```python
from build123d import *

# Parameters (mm, degrees)
SKETCH1_R           = 1.6
BOSS_EXTRUDE1_DEPTH = 2


with BuildPart() as part:
    # Sketch1 → Boss-Extrude1 (new body)
    with BuildSketch(Plane.XY):
        with BuildLine():
            Line((-42, 25.469603275), (-57, 25.469603275))
            Line((-57, 25.469603275), (-57, -22.030396725))
            ThreePointArc((-57, -22.030396725), (-56.121320344, -24.151717068), (-54, -25.030396725))
            Line((-54, -25.030396725), (54, -25.030396725))
            ThreePointArc((54, -25.030396725), (56.121320344, -24.151717068), (57, -22.030396725))
            Line((57, -22.030396725), (57, 25.469603275))
            Line((57, 25.469603275), (42, 25.469603275))
            Line((42, 25.469603275), (42, 55.969603275))
            ThreePointArc((42, 55.969603275), (41.121320344, 58.090923619), (39, 58.969603275))
            Line((39, 58.969603275), (7, 58.969603275))
            Line((7, 58.969603275), (7, 43.469603275))
            Line((7, 43.469603275), (-7, 43.469603275))
            Line((-7, 43.469603275), (-7, 58.969603275))
            Line((-7, 58.969603275), (-39, 58.969603275))
            ThreePointArc((-39, 58.969603275), (-41.121320344, 58.090923619), (-42, 55.969603275))
            Line((-42, 55.969603275), (-42, 25.469603275))
        make_face()
        with Locations((54, -22.030396725)):
            Circle(SKETCH1_R, mode=Mode.SUBTRACT)
        with Locations(Location((-54, -22.030396725, 0), (0, 0, 180))):
            Circle(SKETCH1_R, mode=Mode.SUBTRACT)
        with Locations((39, 55.969603275)):
            Circle(SKETCH1_R, mode=Mode.SUBTRACT)
        with Locations(Location((-39, 55.969603275, 0), (0, 0, 180))):
            Circle(SKETCH1_R, mode=Mode.SUBTRACT)
    extrude(amount=BOSS_EXTRUDE1_DEPTH)


solid = part.part
```
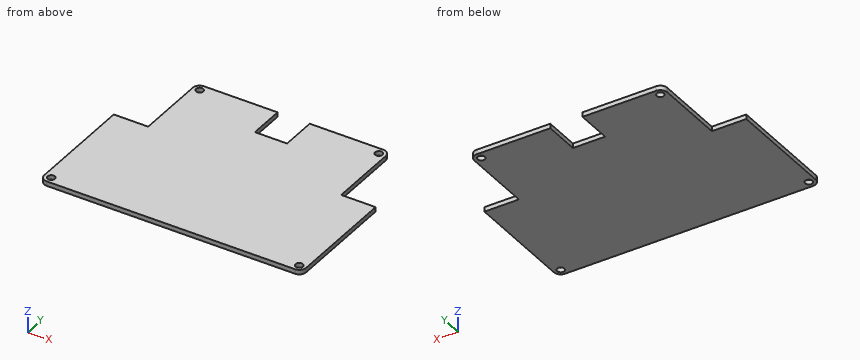
Could you check a few things on this model? Use its own coordinates, in mm. Round coordinates to 2 decimals unless told otherwise and drop trailing zeros. Loops run counter-clockwise (first coordinate to the right, second up) from the corner with the lowest first, then second, coordinate; pieces in that order, holes last. Notation, with made-up numbers: M 44,-4.5 L 93,-4.5 A11 cw 93,1.5 Z; hole C -8.75,56 d2. An arc over 180 degrees is marked long. Answer as CSV lines item,"result".
1) Imagine slicing it at A-A on z = 1. List the corners of the cut face in (x, y) for me, and give its area (3 significant figures).
From the geometry:
outline,"M -57,-22.03 A3 ccw -54,-25.03 L 54,-25.03 A3 ccw 57,-22.03 L 57,25.47 L 42,25.47 L 42,55.97 A3 ccw 39,58.97 L 7,58.97 L 7,43.47 L -7,43.47 L -7,58.97 L -39,58.97 A3 ccw -42,55.97 L -42,25.47 L -57,25.47 Z; hole C -54,-22.03 d3.2; hole C -39,55.97 d3.2; hole C 39,55.97 d3.2; hole C 54,-22.03 d3.2"
area,"8,310 mm^2"
2) If I drill on probe 1 along X at (y, z) = (46, 1.75); probe 2 along Y at (x, z) = (39, 0.8); probe 3 along Y at (x, z) = (54, 1.05), over which ranges is the centre line in solid material (lowest first)?
From the geometry:
probe 1,"-42 to -7, 7 to 42"
probe 2,"-25.03 to 54.37, 57.57 to 58.97"
probe 3,"-25.03 to -23.63, -20.43 to 25.47"
3) For pin 1 Ø0.6 at (y, z) = (54, 1) entering from +X; pin 2 Ø1 at (x, z) = (-3.5, 1) entering from +Y; pin 3 Ø1 at (y, z) = (40, 1.5) entering from -X, each with a flat end and sliding along its axis, tell me the tip position at first contact or that it passes through.
From the geometry:
pin 1,"x = 42"
pin 2,"y = 43.47"
pin 3,"x = -42"
4) Imagine slicing it at B-B on x = 50. List the corners of the cut face in (y, z) for me, and give its area (3 significant figures).
From the geometry:
outline,"M -25.03,0 L 25.47,0 L 25.47,2 L -25.03,2 Z"
area,"101 mm^2"
